from build123d import *

# Parameters (mm, degrees)
BOSS_EXTRUDE1_DEPTH = 20
SKETCH2_R           = 2.95
BOSS_EXTRUDE2_DEPTH = 11
SKETCH4_R           = 2.5
CUT_EXTRUDE1_DEPTH  = 3
SKETCH5_W           = 4
SKETCH5_H           = 2
BOSS_EXTRUDE3_DEPTH = 5


with BuildPart() as part:
    # Sketch1 → Boss-Extrude1 (new body)
    with BuildSketch(Plane.XY):
        Polygon((0, -9), (0, -37), (40, -37), (40, -9), (47, -9), (47, -7), (40, -7), (40, 0), (0, 0), (0, -7), (-7, -7), (-7, -9), align=None)
    extrude(amount=BOSS_EXTRUDE1_DEPTH)

    # Sketch2 → Boss-Extrude2 (add)
    with BuildSketch(Plane(origin=(0, 0, 0), x_dir=(1, 0, 0), z_dir=(0, 1, 0))):
        with Locations(Location((30, -10, 0), (0, 0, 90))):
            Circle(SKETCH2_R)
    extrude(amount=BOSS_EXTRUDE2_DEPTH)

    # Sketch4 → Cut-Extrude1 (cut)
    with BuildSketch(Plane(origin=(0, -7, 0), x_dir=(1, 0, 0), z_dir=(0, 1, 0))):
        with Locations(Location((-4.25, -5, 0), (0, 0, 270))):
            Circle(SKETCH4_R)
        with Locations(Location((-4.25, -15, 0), (0, 0, 270))):
            Circle(SKETCH4_R)
        with Locations(Location((44.25, -5, 0), (0, 0, 270))):
            Circle(SKETCH4_R)
        with Locations(Location((44.25, -15, 0), (0, 0, 270))):
            Circle(SKETCH4_R)
    extrude(amount=-CUT_EXTRUDE1_DEPTH, mode=Mode.SUBTRACT)

    # Sketch5 → Boss-Extrude3 (add)
    with BuildSketch(Plane(origin=(40, 0, 0), x_dir=(0, 0, -1), z_dir=(1, 0, 0))):
        with Locations((-10, -34)):
            Rectangle(SKETCH5_W, SKETCH5_H)
    extrude(amount=BOSS_EXTRUDE3_DEPTH)


solid = part.part
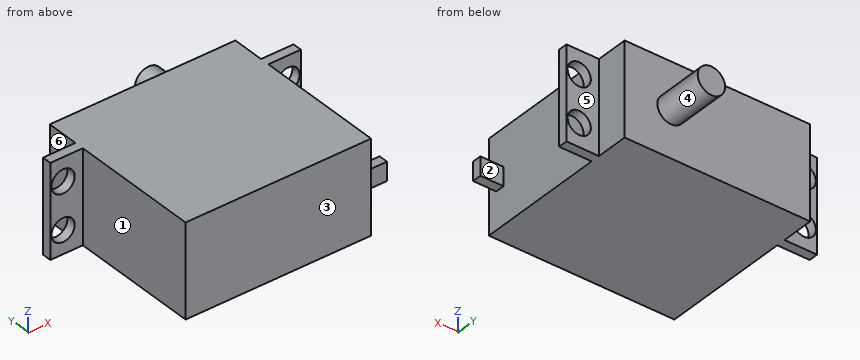
Geometry: final body of the model. Coordinates: model frame, mm. Face numbers are marked on the shaded views. A direction names the side the tool comes from. Give positions to 0.01 mm unless a question says otherwise; leave off trailing zeros. Loops run counter-clockwise (first coordinate to the right, second up) from the corner with the lowest first, then second, coordinate; pieces in that order, holes last. Notation, with made-up numbers: (64.25, 58) -> (119.25, 58) arc R25 ccw to (119.25, 78) -> close; hole circle Ø1 at (-21, 56.5). An arc over 180 degrees is marked (long way). Put each result on its own line as item: value.
1. Pin query (flat end, axial travel): P1, Ø8, axis at x = 33, z = 14, coming from the +Y side; P2, Ø6, axis at x = 12.5, z = 9, coming from the +Y side; P3, Ø2, axis at y = -15.5, z = 2, coming from the +X side; P4, Ø2, axis at x = 31, y = 5, coming from the -Z side. Return the tip coordinate at first contact, or that it passes through.
Taken from the geometry:
P1: stops at y = 11
P2: stops at y = 0
P3: stops at x = 40
P4: stops at z = 7.05
2. Cut plane A-A (z = 15). Return the cut outline in (x, y), plus the area to 3 significant figures.
Taken from the geometry:
outline: (-7, -9) -> (-6.75, -9) -> (-6.75, -7) -> (-7, -7) -> close; (-1.75, -9) -> (0, -9) -> (0, -37) -> (40, -37) -> (40, -9) -> (41.75, -9) -> (41.75, -7) -> (40, -7) -> (40, 0) -> (0, 0) -> (0, -7) -> (-1.75, -7) -> close; (46.75, -9) -> (47, -9) -> (47, -7) -> (46.75, -7) -> close
area: 1,490 mm2
3. Cut plane C-C (z = 10). Return the cut outline in (x, y).
Taken from the geometry:
outline: (-7, -9) -> (0, -9) -> (0, -37) -> (40, -37) -> (40, -35) -> (45, -35) -> (45, -33) -> (40, -33) -> (40, -9) -> (47, -9) -> (47, -7) -> (40, -7) -> (40, 0) -> (32.95, 0) -> (32.95, 11) -> (27.05, 11) -> (27.05, 0) -> (0, 0) -> (0, -7) -> (-7, -7) -> close
4. Ray query, line 1 along Z through (x, y) = (-4, -8); line 2 along X through (y, z) = (-7.9, 5); line 3 along Y through (x, z) = (39.5, 9.5). Return the intervals inside material, ascending. Write a range as [from, to].
Taken from the geometry:
line 1: z = [0, 2.51], [7.49, 12.51], [17.49, 20]
line 2: x = [-7, -6.75], [-1.75, 41.75], [46.75, 47]
line 3: y = [-37, 0]
5. Cut plane B-B (x = 42.5). Return the cut outline in (y, z), plus the area to 3 significant figures.
Taken from the geometry:
outline: (-35, 8) -> (-33, 8) -> (-33, 12) -> (-35, 12) -> close; (-9, 0) -> (-7, 0) -> (-7, 3.21) -> (-9, 3.21) -> close; (-9, 6.79) -> (-7, 6.79) -> (-7, 13.21) -> (-9, 13.21) -> close; (-9, 16.79) -> (-7, 16.79) -> (-7, 20) -> (-9, 20) -> close
area: 33.7 mm2
6. Set-up query: the marked faces 4, 5 and 6. Return all of +Z, -Z, +X, -X, +Y, -Y with unobstructed straight access to the full face (end or side cutting, diameter ignored); none if empty.
Taken from the geometry:
face 4: +Y
face 5: +Z, -Z, +X, +Y
face 6: +Z, -Z, -X, +Y
7. Cut plane D-D (y = -28). Return the cut outline in (x, z).
Taken from the geometry:
outline: (0, 0) -> (40, 0) -> (40, 20) -> (0, 20) -> close
8. Pull-direction query (Y, two-part tool) for the marked faces 1, 2 and 3; classes: released by +Y, released by -Y, zero draft, split by the parting line, or undercut.
Taken from the geometry:
face 1: zero draft
face 2: undercut
face 3: released by -Y
